Source: CAD feature listing. Evaluate the final solid. Frame: model axes, mm. Coordinates: 2 decimals unless noted, no trailing zeros. Order: outer loops, then holes, each group sorted by start corner. A loop starts at its lowest first (then second) coordinate and runs counter-clockwise, first axis right, second up. Notation, with made-up numbers: (45, 16.25) - (58, 16.25) arc R26 ccw to (58, 54.25) - close; hole circle Ø7 at (-38.75, -20). An arc over 180 degrees is marked (long way). One line per question, with ' | ' between items. Start each with the question number.
(1) Section B-B (y = 3.5). Return the cut outline in (x, z).
(2) Section A-A (z = 7.5). Return the cut outline in (x, y), then the cut area to 3 significant figures.
(3) Contact query for a flat-ended pin moving along its axis: P1, Ø8.5, axis at x = 0, z = 6.25, coming from the -Y side. Output: stop coordinate, or through.
(4) Section D-D (z = -1.5). Return the cut outline in (x, y).
(5) Draft query along X for faces 1 (the cylindrical face through (-0.596, 2.685, -6.813)), 2 (the flat face through (8, 0, 0)), 3 (the flat face through (0, 6.35, 0)). Return one class per face: +X half, -X half, draft (parallel to the pull), parting line (faces both ways), or undercut.
(6) Line query: line 1 along X through (y, z) = (0, -8); line 2 along X through (y, z) = (5.25, 6); line 3 along Y through (x, z) = (0, -9.25). Output: solid intervals per line, ascending.
(7) Section C-C (x = 1.25). Return the cut outline in (y, z), then the cut area to 3 significant figures.
from build123d import *

# Parameters (mm, degrees)
F0_W     = 16
F0_H     = 31.5
F1_DEPTH = 6.35
F3_DEPTH = 12.701
F4_R     = 2.75
F5_DEPTH = 31.501


with BuildPart() as f1:
    # F0 (on Front) → F1 (new body, symmetric)
    with BuildSketch(Plane.XZ):
        Rectangle(F0_W, F0_H)
    extrude(amount=F1_DEPTH, both=True)

    # F2 (on face) → F3 (cut, through all)
    with BuildSketch(Plane.XZ.offset(6.35)):
        with BuildLine():
            ThreePointArc((0, 1.5), (3.358757, 2.891243), (4.75, 6.25))
            ThreePointArc((4.75, 6.25), (-3.358757, 9.608757), (0, 1.5))
        make_face()
    extrude(amount=-F3_DEPTH, mode=Mode.SUBTRACT)

    # F4 (on face) → F5 (cut, through all)
    with BuildSketch(Plane(origin=(0, 0, -15.75), x_dir=(1, 0, 0), z_dir=(0, 0, -1))):
        Circle(F4_R)
    extrude(amount=-F5_DEPTH, mode=Mode.SUBTRACT)


solid = f1.part
Response values:
1) outline: (-8, -15.75) - (8, -15.75) - (8, 15.75) - (-8, 15.75) - close; hole circle Ø9.5 at (0, 6.25)
2) outline: (-8, -6.35) - (-4.58, -6.35) - (-4.58, 6.35) - (-8, 6.35) - close; (4.58, -6.35) - (8, -6.35) - (8, 6.35) - (4.58, 6.35) - close | area: 86.8 mm²
3) P1: passes through
4) outline: (-8, -6.35) - (8, -6.35) - (8, 6.35) - (-8, 6.35) - close; hole circle Ø5.5 at (0, 0)
5) face 1: undercut | face 2: +X half | face 3: draft
6) line 1: x = -8 to -2.75, 2.75 to 8 | line 2: x = -8 to -4.74, 4.74 to 8 | line 3: y = -6.35 to -2.75, 2.75 to 6.35
7) outline: (-6.35, -15.75) - (-2.45, -15.75) - (-2.45, 1.67) - (-6.35, 1.67) - close; (-6.35, 10.83) - (-2.45, 10.83) - (-2.45, 15.75) - (-6.35, 15.75) - close; (2.45, -15.75) - (6.35, -15.75) - (6.35, 1.67) - (2.45, 1.67) - close; (2.45, 10.83) - (6.35, 10.83) - (6.35, 15.75) - (2.45, 15.75) - close | area: 174 mm²
